```python
from build123d import *

# Parameters (mm, degrees)
SKETCH1_R           = 3.429
SKETCH1_R_2         = 2.54
BOSS_EXTRUDE1_DEPTH = 3.2004
SKETCH2_R           = 1.7272
CUT_EXTRUDE1_DEPTH  = 3.2004
SKETCH5_R           = 1.7272
SKETCH5_W           = 40.894
SKETCH5_H           = 20.32
CUT_EXTRUDE3_DEPTH  = 4.2004
CUT_EXTRUDE4_DEPTH  = 3.2004
SKETCH8_R           = 1.7272
CUT_EXTRUDE6_DEPTH  = 3.2004
SKETCH9_R           = 1.7272
SKETCH9_R_2         = 2.54
SKETCH9_W           = 40.894
SKETCH9_H           = 20.32
CUT_EXTRUDE8_DEPTH  = 3.2004
CUT_EXTRUDE9_DEPTH  = 3.2004
FILLET1_R           = 5.08
SKETCH11_R          = 2.159
CUT_EXTRUDE10_DEPTH = 3.2004
CUT_EXTRUDE11_DEPTH = 3.2004
SKETCH13_R          = 13.885201093
CUT_EXTRUDE12_DEPTH = 3.2004
SKETCH14_R          = 2.54
CUT_EXTRUDE13_DEPTH = 3.2004
CUT_EXTRUDE14_DEPTH = 3.2004
FILLET2_R           = 12.7


with BuildPart() as part:
    # Sketch1 → Boss-Extrude1 (new body)
    with BuildSketch(Plane.XY):
        with BuildLine():
            Line((0, 0), (120.015, 0))
            ThreePointArc((120.015, 0), (130.351788396, 3.075697789), (137.325636158, 11.302152592))
            Line((137.325636158, 11.302152592), (155.2575, 52.11572))
            ThreePointArc((155.2575, 52.11572), (157.08610336, 70.335755455), (147.862829504, 86.154880008))
            ThreePointArc((147.862829504, 86.154880008), (60.0075, 119.675648416), (-27.847829504, 86.154880008))
            ThreePointArc((-27.847829504, 86.154880008), (-37.07110336, 70.335755455), (-35.2425, 52.11572))
            Line((-35.2425, 52.11572), (-17.310636158, 11.302152592))
            ThreePointArc((-17.310636158, 11.302152592), (-10.336788396, 3.075697789), (0, 0))
        make_face()
        with Locations((120.015, 18.90776)):
            Circle(SKETCH1_R, mode=Mode.SUBTRACT)
        with Locations((0, 18.90776)):
            Circle(SKETCH1_R, mode=Mode.SUBTRACT)
        with Locations((19.734727626, 25.566426992)):
            Circle(SKETCH1_R_2, mode=Mode.SUBTRACT)
    extrude(amount=BOSS_EXTRUDE1_DEPTH)

    # Sketch2 → Cut-Extrude1 (cut)
    with BuildSketch(Plane(origin=(0, 0, 0), x_dir=(-1, 0, 0), z_dir=(0, 0, -1))):
        with Locations((-92.0115, 52.11572)):
            Circle(SKETCH2_R)
        with Locations((-76.0095, 52.11572)):
            Circle(SKETCH2_R)
        with Locations((-44.0055, 52.11572)):
            Circle(SKETCH2_R)
        with Locations((-28.0035, 52.11572)):
            Circle(SKETCH2_R)
    extrude(amount=-CUT_EXTRUDE1_DEPTH, mode=Mode.SUBTRACT)

    # Sketch5 → Cut-Extrude3 (cut, through all)
    with BuildSketch(Plane(origin=(0, 0, 0), x_dir=(-1, 0, 0), z_dir=(0, 0, -1))):
        with Locations((-79.746999972, 23.90776)):
            Circle(SKETCH5_R)
        with Locations((-29.246999972, 13.90776)):
            Circle(SKETCH5_R)
        with Locations((-29.246999972, 23.90776)):
            Circle(SKETCH5_R)
        with Locations((-79.746999972, 13.90776)):
            Circle(SKETCH5_R)
        with Locations((-92.322240346, 23.90776)):
            Circle(SKETCH5_R)
        with Locations((-92.322240346, 13.90776)):
            Circle(SKETCH5_R)
        with Locations((-54.496999972, 18.90776)):
            Rectangle(SKETCH5_W, SKETCH5_H)
    extrude(amount=-CUT_EXTRUDE3_DEPTH, mode=Mode.SUBTRACT)

    # Sketch6 → Cut-Extrude4 (cut)
    with BuildSketch(Plane.XY.offset(3.2004)):
        with BuildLine():
            Line((29.985999972, 19.92376), (34.049999972, 19.92376))
            Line((34.049999972, 19.92376), (34.049999972, 17.89176))
            Line((34.049999972, 17.89176), (29.985999972, 17.89176))
            ThreePointArc((29.985999972, 17.89176), (28.969999972, 18.90776), (29.985999972, 19.92376))
        make_face()
        with BuildLine():
            Line((74.943999972, 19.92376), (79.007999972, 19.92376))
            ThreePointArc((79.007999972, 19.92376), (80.023999972, 18.90776), (79.007999972, 17.89176))
            Line((79.007999972, 17.89176), (74.943999972, 17.89176))
            Line((74.943999972, 17.89176), (74.943999972, 19.92376))
        make_face()
    extrude(amount=-CUT_EXTRUDE4_DEPTH, mode=Mode.SUBTRACT)

    # Sketch8 → Cut-Extrude6 (cut)
    with BuildSketch(Plane.XY.offset(3.2004)):
        with Locations((21.9075, 3.81)):
            Circle(SKETCH8_R)
        with Locations((60.0075, 3.81)):
            Circle(SKETCH8_R)
        with Locations((98.1075, 3.81)):
            Circle(SKETCH8_R)
    extrude(amount=-CUT_EXTRUDE6_DEPTH, mode=Mode.SUBTRACT)

    # Sketch9 → Cut-Extrude8 (cut)
    with BuildSketch(Plane(origin=(0, 0, 0), x_dir=(-1, 0, 0), z_dir=(0, 0, -1))):
        with Locations((-105.391483991, 85.535782838)):
            Circle(SKETCH9_R)
        with Locations((-105.860285109, 92.437383775)):
            Circle(SKETCH9_R_2)
        with Locations((-54.891483991, 75.535782838)):
            Circle(SKETCH9_R)
        with Locations((-54.891483991, 85.535782838)):
            Circle(SKETCH9_R)
        with Locations((-105.391483991, 75.535782838)):
            Circle(SKETCH9_R)
        with Locations((-126.474462623, 80.535782838)):
            Circle(SKETCH9_R_2)
        with Locations((-80.141483991, 80.535782838)):
            Rectangle(SKETCH9_W, SKETCH9_H)
    extrude(amount=-CUT_EXTRUDE8_DEPTH, mode=Mode.SUBTRACT)

    # Sketch10 → Cut-Extrude9 (cut)
    with BuildSketch(Plane.XY.offset(3.2004)):
        with BuildLine():
            Line((-24.96979716, 88.651483667), (-19.207398738, 77.007598217))
            Line((-19.207398738, 77.007598217), (26.33351958, 99.545171003))
            Line((26.33351958, 99.545171003), (35.569015789, 117.391739689))
            ThreePointArc((35.569015789, 117.391739689), (3.443784755, 106.930742334), (-24.96979716, 88.651483667))
        make_face()
    extrude(amount=-CUT_EXTRUDE9_DEPTH, mode=Mode.SUBTRACT)

    # Fillet1
    fillet1_edges = [part.edges().sort_by_distance(p)[0] for p in [
        (35.569015789, 117.391739689, 1.6002),
        (-24.96979716, 88.651483667, 1.6002),
    ]]
    fillet(fillet1_edges, radius=FILLET1_R)

    # Sketch11 → Cut-Extrude10 (cut)
    with BuildSketch(Plane(origin=(0, 0, 0), x_dir=(-1, 0, 0), z_dir=(0, 0, -1))):
        with Locations((-32.004, 70.53072)):
            Circle(SKETCH11_R)
        with Locations((-24.003, 70.53072)):
            Circle(SKETCH11_R)
        with BuildLine():
            Line((-34.3535, 80.05572), (-21.6535, 80.05572))
            ThreePointArc((-21.6535, 80.05572), (-18.4785, 76.88072), (-21.6535, 73.70572))
            Line((-21.6535, 73.70572), (-34.3535, 73.70572))
            ThreePointArc((-34.3535, 73.70572), (-37.5285, 76.88072), (-34.3535, 80.05572))
        make_face()
    extrude(amount=-CUT_EXTRUDE10_DEPTH, mode=Mode.SUBTRACT)

    # Sketch12 → Cut-Extrude11 (cut)
    with BuildSketch(Plane(origin=(0, 0, 0), x_dir=(-1, 0, 0), z_dir=(0, 0, -1))):
        with BuildLine():
            Line((-104.652483991, 81.551782838), (-100.588483991, 81.551782838))
            Line((-100.588483991, 81.551782838), (-100.588483991, 79.519782838))
            Line((-100.588483991, 79.519782838), (-104.652483991, 79.519782838))
            ThreePointArc((-104.652483991, 79.519782838), (-105.668483991, 80.535782838), (-104.652483991, 81.551782838))
        make_face()
        with BuildLine():
            Line((-59.694483991, 81.551782838), (-55.630483991, 81.551782838))
            ThreePointArc((-55.630483991, 81.551782838), (-54.614483991, 80.535782838), (-55.630483991, 79.519782838))
            Line((-55.630483991, 79.519782838), (-59.694483991, 79.519782838))
            Line((-59.694483991, 79.519782838), (-59.694483991, 81.551782838))
        make_face()
    extrude(amount=-CUT_EXTRUDE11_DEPTH, mode=Mode.SUBTRACT)

    # Sketch13 → Cut-Extrude12 (cut)
    with BuildSketch(Plane(origin=(0, 0, 0), x_dir=(-1, 0, 0), z_dir=(0, 0, -1))):
        with Locations((-49.53, 18.90776)):
            Circle(SKETCH13_R)
    extrude(amount=-CUT_EXTRUDE12_DEPTH, mode=Mode.SUBTRACT)

    # Sketch14 → Cut-Extrude13 (cut)
    with BuildSketch(Plane(origin=(0, 0, 0), x_dir=(-1, 0, 0), z_dir=(0, 0, -1))):
        with Locations((-99.400822485, 30.809360937)):
            Circle(SKETCH14_R)
    extrude(amount=-CUT_EXTRUDE13_DEPTH, mode=Mode.SUBTRACT)

    # Sketch15 → Cut-Extrude14 (cut)
    with BuildSketch(Plane(origin=(0, 0, 0), x_dir=(-1, 0, 0), z_dir=(0, 0, -1))):
        Polygon((33.771104783, 106.435991135), (93.302614335, 68.041010777), (77.912627241, 47.955189764), (19.207398738, 77.007598217), align=None)
    extrude(amount=-CUT_EXTRUDE14_DEPTH, mode=Mode.SUBTRACT)

    # Fillet2
    fillet2_edges = [part.edges().sort_by_distance(p)[0] for p in [
        (-37.48662973, 67.961458741, 1.6002),
    ]]
    fillet(fillet2_edges, radius=FILLET2_R)


solid = part.part
```
Geometry: final body of the model. Coordinates: model frame, mm. A direction names the side the tool comes from. Round coordinates to 2 decimals unless told otherwise and drop trailing zeros. Write each loop counter-clockwise with the first axis right and the second up, starting at its lowest first coordinate (ties: lowest second). Pieces come first, ordered by that corner, then holes. Notation, with made-up numbers: (77, 59) -> (91, 59) arc R33 ccw to (91, 91) -> close; hole circle Ø1 at (-5, 58). An arc over 180 degrees is marked (long way). Return JSON: item names as keys, results as strings.
Q1. Section A-A on z = 0.75. Give the number of separate pieces and of enclosed holes in the cut face, and give its area (3 significant figures).
From the geometry:
{"separate pieces": "1", "enclosed holes": "28", "area": "15,800 mm2"}
Q2. Ray query, line 1 (Y direction, x = 25.5, z = 0.2) (3 decimals); line 2 (Y direction, x = 25, z = 0.7); line 3 (X direction, y = 90.5, z = 2.65). Return the intervals inside material, ascending.
From the geometry:
{"line 1": "0 to 68.975, 72.086 to 73.706, 80.056 to 99.133", "line 2": "0 to 68.62, 72.45 to 73.71, 80.06 to 98.89", "line 3": "8.06 to 59.69, 100.59 to 104.22, 107.5 to 142.74"}
Q3. First-contact query: pin 1 Ø1 at (y, z) = (99, 1) entering from +X; pin 2 Ø1 at (x, z) = (85.5, 2) entering from +Y; pin 3 Ø1.6 at (y, z) = (14, 2.5) entering from +X. Flat tips, straight axial feed; report the tip coordinate or a pass-through.
From the geometry:
{"pin 1": "x = 131.68", "pin 2": "y = 117.29", "pin 3": "x = 138.86"}
Q4. Set-up query: faces 1 (the cylindrical face through (49.676, 5.023, 1.578)), 2 (the cylindrical face through (97.38, 114.27, 1.58)). Return all of +Z, -Z, +X, -X, +Y, -Y with unobstructed straight access to the full face (end or side cutting, diameter ignored); none if empty.
From the geometry:
{"face 1": "+Z, -Z", "face 2": "+Z, -Z, +Y"}
Q5. Section B-B on x = 134. Return the cut outline in (y, z), and give its area (3 significant figures).
From the geometry:
{"outline": "(6.18, 0) -> (96.97, 0) -> (96.97, 3.2) -> (6.18, 3.2) -> close", "area": "291 mm2"}
Q6. Section C-C on x = -12.5. Return the cut outline in (y, z).
From the geometry:
{"outline": "(4.72, 0) -> (80.33, 0) -> (80.33, 3.2) -> (4.72, 3.2) -> close"}
Q7. Mould query, pull axis X, two halves, no side actions, for faces 3 (the cylindrical face through (77.38, 51.065, 1.578)), 4 (the flat face through (-26.4, 31.99, 1.58)), 5 (the flat face through (59, 61, 3.2)). Classes: +X half, -X half, draft (parallel to the pull), parting line (faces both ways), or undercut.
From the geometry:
{"face 3": "undercut", "face 4": "-X half", "face 5": "draft"}
